Here's the drawing with two shaded views (mm, measured from the low corner). I have some questions. Coordinates: 2 decimals unless noted, no trailing zeros. Loops run counter-clockwise (first coordinate to the right, second up) from the corner with the lowest first, then second, coordinate; pieces in that order, holes last. Notation, with made-up numbers: (87, -13.5) - (136, -13.5) arc R11 cw to (136, -0.5) - close; hole circle Ø1 at (48.25, -17). An arc over 180 degrees is marked (long way). One line per item, written item: value. Start each with the question number.
(1) If we section it at A-A on x = 254: Write out the boundary of the cut face in (y, z).
(2) I'm going to push a flat-ended pin straight in: P1, Ø6, axis at y = 16.5, z = 249.5, coming from the -X side. Where does the tip first touch, or does it pass through?
(3) If I drill on line 1 along X through (y, z) = (10.25, 667.5); line 2 along Z through (x, y) = (280, 2.5); line 3 along Z through (x, y) = (273.5, 11.75), over which ranges is the centre line in solid material (lowest first)? Write a range as from..to.
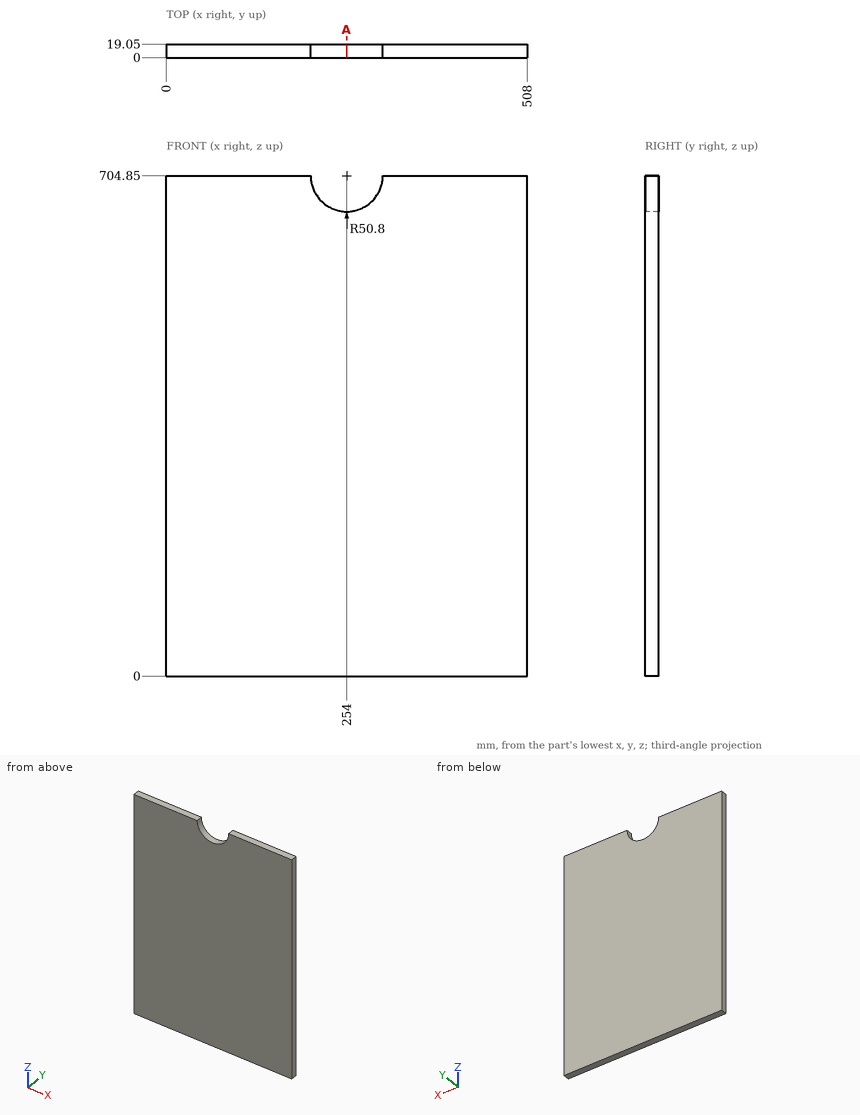
Values:
1. outline: (0, 0) - (19.05, 0) - (19.05, 654.05) - (0, 654.05) - close
2. P1: stops at x = 0
3. line 1: x = 0..219.57, 288.43..508
3. line 2: z = 0..661.21
3. line 3: z = 0..657.94
